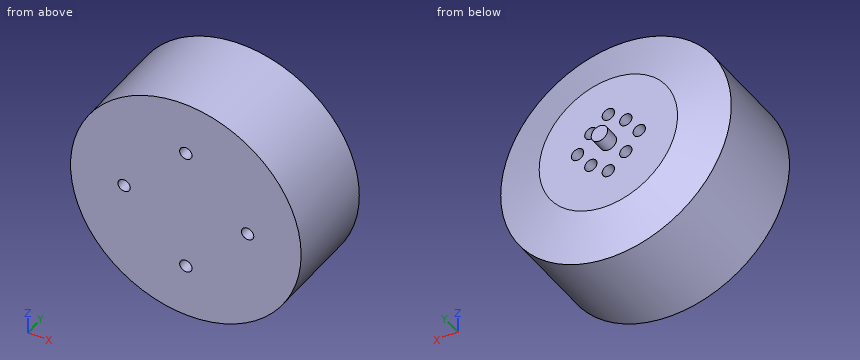
```python
from build123d import *

# Parameters (mm, degrees)
SKETCH1_R           = 28
BOSS_EXTRUDE1_DEPTH = 25.8
SKETCH2_R           = 2
BOSS_EXTRUDE2_DEPTH = 3.5
SKETCH3_R           = 1.5
CUT_EXTRUDE1_DEPTH  = 3
SKETCH4_R           = 1.5
CUT_EXTRUDE2_DEPTH  = 3
CHAMFER1_SIZE       = 3
CHAMFER1_SIZE2      = 11.196152423


with BuildPart() as part:
    # Sketch1 → Boss-Extrude1 (new body)
    with BuildSketch(Plane(origin=(0, 0, 0), x_dir=(1, 0, 0), z_dir=(0, 1, 0))):
        Circle(SKETCH1_R)
    extrude(amount=BOSS_EXTRUDE1_DEPTH)

    # Sketch2 → Boss-Extrude2 (add)
    with BuildSketch(Plane(origin=(0, 25.8, 0), x_dir=(1, 0, 0), z_dir=(0, 1, 0))):
        Circle(SKETCH2_R)
    extrude(amount=BOSS_EXTRUDE2_DEPTH)

    # Sketch3 → Cut-Extrude1 (cut)
    with BuildSketch(Plane.XZ):
        with Locations((0, 15)):
            Circle(SKETCH3_R)
        with Locations((15, 0)):
            Circle(SKETCH3_R)
        with Locations((0, -15)):
            Circle(SKETCH3_R)
        with Locations((-15, 0)):
            Circle(SKETCH3_R)
    extrude(amount=-CUT_EXTRUDE1_DEPTH, mode=Mode.SUBTRACT)

    # Sketch4 → Cut-Extrude2 (cut)
    with BuildSketch(Plane(origin=(0, 25.8, 0), x_dir=(1, 0, 0), z_dir=(0, 1, 0))):
        with Locations((0, 7.5)):
            Circle(SKETCH4_R)
        with Locations((7.5, 0)):
            Circle(SKETCH4_R)
        with Locations((0, -7.5)):
            Circle(SKETCH4_R)
        with Locations((-7.5, 0)):
            Circle(SKETCH4_R)
        with Locations((4.242640687, 4.242640687)):
            Circle(SKETCH4_R)
        with Locations((4.242640687, -4.242640687)):
            Circle(SKETCH4_R)
        with Locations((-4.242640687, -4.242640687)):
            Circle(SKETCH4_R)
        with Locations((-4.242640687, 4.242640687)):
            Circle(SKETCH4_R)
    extrude(amount=-CUT_EXTRUDE2_DEPTH, mode=Mode.SUBTRACT)

    # Chamfer1
    chamfer1_edges = [part.edges().sort_by_distance(p)[0] for p in [
        (-28, 25.8, 0),
    ]]
    chamfer1_side = [part.faces().sort_by_distance(p)[0] for p in [
        (-28, 12.9, 0),
    ]]
    chamfer(chamfer1_edges, length=CHAMFER1_SIZE, length2=CHAMFER1_SIZE2, reference=chamfer1_side[0])


solid = part.part
```
Model file for the job. Use its own axes, mm. Coordinates: 2 decimals unless noted, no trailing zeros. Loops run counter-clockwise (first coordinate to the right, second up) from the corner with the lowest first, then second, coordinate; pieces in that order, holes last. Notation, with made-up numbers: (47.25, 20) -> (52.25, 20) arc R20 cw to (52.25, 33) -> close; hole circle Ø11 at (-33, 47.5). An arc over 180 degrees is marked (long way). Answer as a JSON object with one key per item and string values.
Q1. Flat gauge pins, fed straight in: P1, Ø1.5, axis at x = 0.5, z = 7.5, coming from the +Y side; P2, Ø0.9, axis at x = 0, z = -15, coming from the -Y side; P3, Ø8, axis at y = 22, z = 21.5, coming from the -X side. Where does each tip first touch, or does it go through?
Report:
{"P1": "stops at y = 22.8", "P2": "stops at y = 3", "P3": "stops at x = -21.86"}
Q2. Probe probe 1 along Z at (x, y) = (0, 1.85); probe 2 along Y at (x, z) = (-1, 13); probe 3 along Y at (x, z) = (15, 20.5). List the from-to ranges inside material, lowest first.
Report:
{"probe 1": "z = -28 to -16.5, -13.5 to 13.5, 16.5 to 28", "probe 2": "y = 0 to 25.8", "probe 3": "y = 0 to 23.5"}
Q3. Cut at A-A (y = 15). List the corners of the cut face in (x, z), and give its area (3 significant figures).
Report:
{"outline": "circle Ø56 at (0, 0)", "area": "2,460 mm2"}
